Read the model definition and answer for the solid it produces. Units are mm, in the model's axes. Give positions to 0.01 mm unless a question says otherwise; leave off trailing zeros. Loops run counter-clockwise (first coordinate to the right, second up) from the corner with the lowest first, then second, coordinate; pieces in that order, holes last. Notation, with made-up numbers: (-14.5, -37.5) -> (-1.5, -37.5) arc R35 cw to (-1.5, 0.5) -> close; hole circle Ø2 at (-25, 1). An arc over 180 degrees is marked (long way). Write each question's results on one line, items separated by ' | '. Start each with the question number.
Item 1: This flat-tipped pin is pushed along its axis until it touches: P1, Ø5, axis at x = 0, y = 0, coming from the -Z side. Where does it stop, or does it pass through?
Item 2: Section A-A on y = 0 is taken. Write down the section's boundary in (x, z) (3 decimals).
Item 3: Determine the mould class of faces 1 (the cylindrical face through (-3.8, -1.6, 0.5)), 2 (the flat face through (0, -5, 0)), 3 (the cylindrical face through (2.38, -10.74, 0.49)) for opening direction X: +X half, -X half, draft (parallel to the pull), parting line (faces both ways), or undercut.
Item 4: Section D-D on y = -4.75 is taken. Write down the section's boundary in (x, z).
Item 5: Find the intervals of material crossed by line 1 (Y direction, x = 0, z = 0.75) (3 decimals); line 2 (Y direction, x = -3.5, z = 0.15); line 3 (X direction, y = -1, z = 0.4), in increasing order.
Item 6: Section C-C on z = 0.4 is taken. Write down the section's boundary in (x, y) (3 decimals), and give its area (3 significant figures).
Autodesk Inventor part; units mm, degrees
ref_plane "YZ Plane" through (0, 0, 0) normal (1, 0, 0) x (0, 1, 0)
ref_plane "XZ Plane" through (0, 0, 0) normal (0, 1, 0) x (-1, 0, 0)
ref_plane "XY Plane" through (0, 0, 0) normal (0, 0, 1) x (1, 0, 0)
sketch "スケッチ1" plane through (0, 0, 0) normal (0, 0, 1) x (1, 0, 0)
  circle A0 centre (0, 0) radius 3.125
  circle A1 centre (0, 0) radius 6
  dimension "d0" = 6.25
  dimension "d1" = 12
extrude "押し出し1" add sketch "スケッチ1" along normal blind 1
sketch "스케치2" plane through (0, 0, 0) normal (0, 0, -1) x (-1, 0, 0)
  circle A0 centre (0, 0) radius 6
  circle A1 centre (0, 0) radius 3.125
  circle A2 centre (0, 0) radius 4.125
  dimension "d4" = 8.25
extrude "돌출2" cut sketch "스케치2" against normal through all contours A2
sketch "스케치3" plane through (0, 0, 0) normal (0, 0, -1) x (-1, 0, 0)
  circle A0 centre (0, 0) radius 4.125
  circle A1 centre (0, 0) radius 6
  circle A2 centre (0, 0) radius 11
  dimension "d7" = 22
extrude "돌출3" add sketch "스케치3" against normal blind 1 contours A2
properties part number "TT-0822-10" material "PET プラスチック"
Findings:
1) P1: through
2) outline: (-11, 0) -> (-4.125, 0) -> (-4.125, 1) -> (-11, 1) -> close; (4.125, 0) -> (11, 0) -> (11, 1) -> (4.125, 1) -> close
3) face 1: undercut | face 2: draft | face 3: parting line
4) outline: (-9.92, 0) -> (9.92, 0) -> (9.92, 1) -> (-9.92, 1) -> close
5) line 1: -11 to -4.125, 4.125 to 11 | line 2: -10.43 to -2.18, 2.18 to 10.43 | line 3: -10.95 to -4, 4 to 10.95
6) outline: circle Ø22 at (0, 0); hole circle Ø8.25 at (0, 0) | area: 327 mm2
